Part model, mm, in its own coordinate system. A direction names the side the tool comes from. Round coordinates to 2 decimals unless told otherwise and drop trailing zeros. Order: outer loops, then holes, each group sorted by start corner. A loop starts at its lowest first (then second) coordinate and runs counter-clockwise, first axis right, second up. Notation, with made-up numbers: (79, -24) -> (94, -24) arc R12 ccw to (94, -9) -> close; hole circle Ø2 at (46, -16). An arc over 180 degrees is marked (long way). Answer as a JSON object with one key per item and string values. Group by question number.
```python
from build123d import *

# Parameters (mm, degrees)
SKETCH1_W           = 25.4
SKETCH1_H           = 3.175
BOSS_EXTRUDE1_DEPTH = 6.35
SKETCH2_R           = 2.4003
CUT_EXTRUDE1_DEPTH  = 8.89
FILLET1_R           = 0.635
CUT_EXTRUDE2_DEPTH  = 3.81


with BuildPart() as part:
    # Sketch1 → Boss-Extrude1 (new body)
    with BuildSketch(Plane(origin=(0, 0, 0), x_dir=(1, 0, 0), z_dir=(0, 1, 0))):
        with Locations((12.7, 4.7625)):
            Rectangle(SKETCH1_W, SKETCH1_H)
        with Locations((12.7, 1.5875)):
            Rectangle(SKETCH1_W, SKETCH1_H)
        Polygon((25.4, 6.35), (25.4, 3.175), (38.1, 3.175), (25.4, 9.525), align=None)
        Polygon((38.1, 3.175), (25.4, 3.175), (25.4, 0), (25.4, -3.175), align=None)
    extrude(amount=BOSS_EXTRUDE1_DEPTH)

    # Sketch2 → Cut-Extrude1 (cut)
    with BuildSketch(Plane.ZY):
        with Locations((-3.175, 3.175)):
            Circle(SKETCH2_R)
    extrude(amount=-CUT_EXTRUDE1_DEPTH, mode=Mode.SUBTRACT)

    # Fillet1
    fillet1_edges = [part.edges().sort_by_distance(p)[0] for p in [
        (0, 3.175, -6.35),
        (25.4, 3.175, -6.35),
        (25.4, 3.175, -9.525),
        (38.1, 3.175, -3.175),
        (25.4, 3.175, 3.175),
        (25.4, 3.175, 0),
        (0, 3.175, 0),
    ]]
    fillet(fillet1_edges, radius=FILLET1_R)

    # Sketch3 → Cut-Extrude2 (cut)
    with BuildSketch(Plane.XZ):
        with BuildLine():
            ThreePointArc((11.926548417, -3.175), (11.037548417, -2.286), (10.148548417, -3.175))
            Line((10.148548417, -3.175), (11.926548417, -3.175))
        make_face()
        with BuildLine():
            Line((11.926548417, -3.175), (10.148548417, -3.175))
            ThreePointArc((10.148548417, -3.175), (11.037548417, -4.064), (11.926548417, -3.175))
        make_face()
        with BuildLine():
            ThreePointArc((27.166548417, -3.175), (26.277548417, -2.286), (25.388548417, -3.175))
            Line((25.388548417, -3.175), (27.166548417, -3.175))
        make_face()
        with BuildLine():
            Line((27.166548417, -3.175), (25.388548417, -3.175))
            ThreePointArc((25.388548417, -3.175), (26.277548417, -4.064), (27.166548417, -3.175))
        make_face()
    extrude(amount=-CUT_EXTRUDE2_DEPTH, mode=Mode.SUBTRACT)


solid = part.part
```
Q1. Band-saw the part on B-B (y = 2.75). Count the separate pieces of the cut face and the enclosed holes in it, plus the area to 3 significant figures.
Q2. Which spindle directions (+Z, -Z, +X, -X, +Y, -Y) get a long thin tool onto all of the face, cutting with end or side? Do faces 4 (the flat face through (8.89, 3, -3)), 5 (the flat face through (26, 3.81, -3)), 6 (the flat face through (13, 3, 0)), 7 (the flat face through (13, 3, -6.35)). Say none if no direction does.
Q3. Wall check: line 1 (Z direction, x = 3, y = 3); line 2 (X direction, y = 2.5, z = -3.75); line 3 (Z direction, x = 11, y = 0.5). Give the ranges that are in metal, low to high. Write a range as [from, to].
Q4. Two-plate mould, pull along Y, no slides. Class faces 1 (the cylindrical face through (4.383, 3.896, -0.886)), 2 (the flat face through (18, 0, -3)), 3 (the cylindrical face through (37.315, 3.219, -3.165)): +Y half, -Y half, draft (parallel to the pull), parting line (faces both ways), or undercut.
Q5. Band-saw the part on C-C (x = 3.5). List the corners of the cut face in (y, z) (3 decimals), plus the area to 3 significant figures.
Q6. Drop flat-ended pins along their axis: pin 1 Ø1.4 at (y, z) = (2.5, -3) entering from -X; pin 2 Ø3 at (x, y) = (8.5, 4) entering from +Z; pin 3 Ø1.2 at (y, z) = (3, 1.5) entering from -X. Give the stop position or say it passes through.
Q7. Band-saw the part on A-A (z = -5). List the corners of the cut face in (x, y).
Q8. Band-saw the part on D-D (x = 21.5). List the corners of the cut face in (y, z).
Completed:
{
 "1": {"separate pieces": "1", "enclosed holes": "2", "area": "194 mm2"},
 "2": {"face 4": "-X", "face 5": "-Y", "face 6": "+Z, -X, +Y, -Y", "face 7": "-Z, -X, +Y, -Y"},
 "3": {"line 1": "[-6.35, -5.57], [-0.78, 0]", "line 2": "[8.89, 10.36], [11.72, 25.6], [26.96, 36.95]", "line 3": "[-6.35, -4.06], [-2.29, 0]"},
 "4": {"face 1": "undercut", "face 2": "-Y half", "face 3": "draft"},
 "5": {"outline": "(0, -6.35) -> (6.35, -6.35) -> (6.35, 0) -> (0, 0) -> close; hole circle Ø4.801 at (3.175, -3.175)", "area": "22.2 mm2"},
 "6": {"pin 1": "x = 8.89", "pin 2": "z = 0", "pin 3": "x = 25.4"},
 "7": {"outline": "(0, 0) -> (34.45, 0) -> (34.45, 6.35) -> (0, 6.35) -> (0, 4.73) -> (8.89, 4.73) -> (8.89, 1.62) -> (0, 1.62) -> close"},
 "8": {"outline": "(0, -6.35) -> (6.35, -6.35) -> (6.35, 0) -> (0, 0) -> close"}
}
